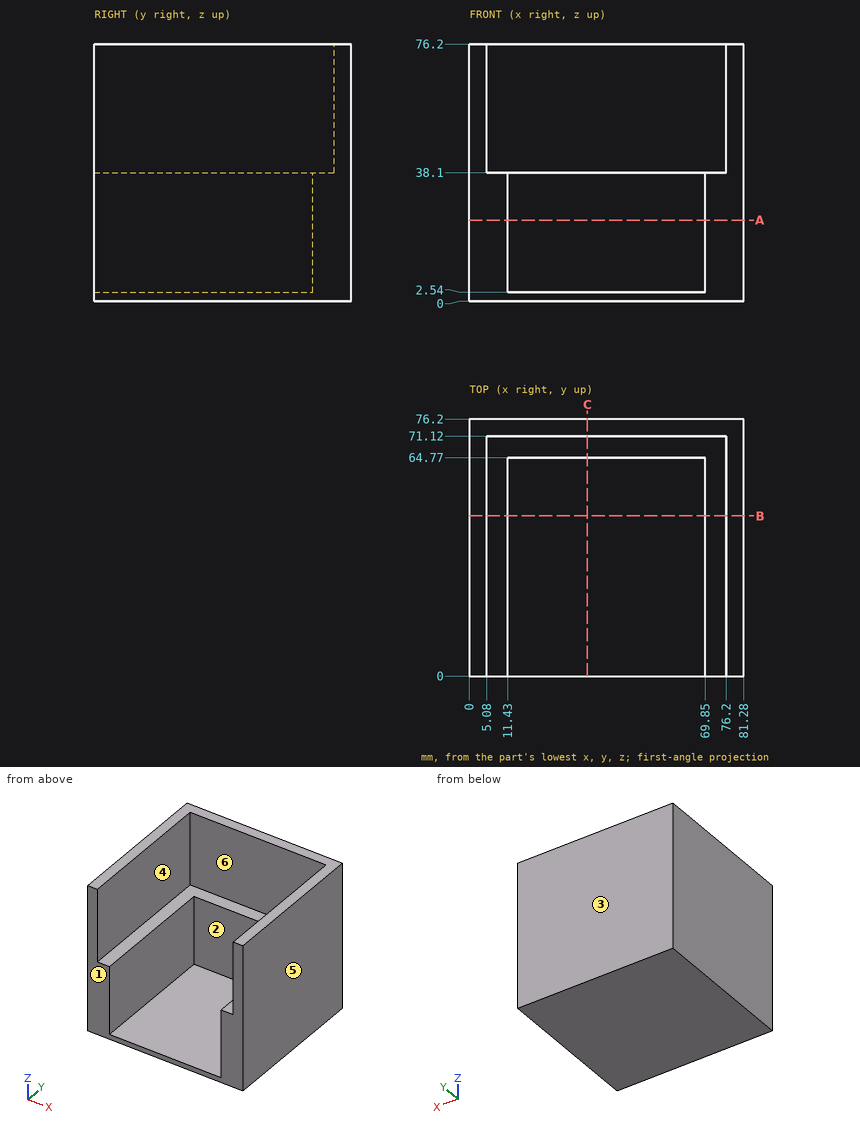
The figure shows three views and two pictorial views of one solid part (mm, origin at its lowest corner). Answer the questions. A direction names the side the tool comes from. Round coordinates to 2 decimals unless told otherwise and drop trailing zeros. Order: outer loops, then holes, each group sorted by start corner. A loop starts at its lowest first (then second) coordinate and runs counter-clockwise, first axis right, second up.
Q1. Find the intervals of material crossed by line 1 along X through (y, z) = (52.5, 57); line 2 along X through (y, z) = (24.5, 7); line 3 along Z through (x, y) = (17, 51.5), in increasing order.
Solution:
line 1: x = 0 to 5.08, 76.2 to 81.28
line 2: x = 0 to 11.43, 69.85 to 81.28
line 3: z = 0 to 2.54
Q2. The mould has two halves that part along X. Classify the marked faces 3, 4, 5 and 6: pulls with the +X half, pulls with the -X half, needs draft (parallel to the pull), parting line crosses it, or undercut.
Solution:
face 3: needs draft
face 4: undercut
face 5: pulls with the +X half
face 6: undercut
Q3. Given pin 1 Ø5 at (x, y) = (55, 17) entering from +Z; pin 2 Ø11.5 at (x, z) = (33.5, 62.5) entering from -Y; pin 3 Ø4 at (x, y) = (70.5, 48) entering from +Z, each flat-ended and moving along its own axis, determine where each tip first touches the part or whether it passes through.
Solution:
pin 1: stops at z = 2.54
pin 2: stops at y = 71.12
pin 3: stops at z = 38.1
Q4. A tool of negligible diameter and unlimited length cuts with its end or side. For the marked faces 1 and 2, from which of +Z, -Z, +X, -X, +Y, -Y can it reach the whole face along a straight path? Write none if from no direction.
Solution:
face 1: +Z, -Z, +X, -X, -Y
face 2: +Z, -Y
Q5. A cutting plane is placed at A-A, the plane z = 24. Determine the outline of the cut face in (x, y).
Solution:
outline: (0, 0) - (11.43, 0) - (11.43, 64.77) - (69.85, 64.77) - (69.85, 0) - (81.28, 0) - (81.28, 76.2) - (0, 76.2) - close
Q6. A cutting plane is placed at B-B, the plane y = 47.5. Determine the outline of the cut face in (x, z).
Solution:
outline: (0, 0) - (81.28, 0) - (81.28, 76.2) - (76.2, 76.2) - (76.2, 38.1) - (69.85, 38.1) - (69.85, 2.54) - (11.43, 2.54) - (11.43, 38.1) - (5.08, 38.1) - (5.08, 76.2) - (0, 76.2) - close
Q7. A cutting plane is placed at C-C, the plane x = 35. Determine the outline of the cut face in (y, z).
Solution:
outline: (0, 0) - (76.2, 0) - (76.2, 76.2) - (71.12, 76.2) - (71.12, 38.1) - (64.77, 38.1) - (64.77, 2.54) - (0, 2.54) - close
